Source: three-view drawing plus pictorial views. Frame: mm from the lowest corner of the part. A direction names the side the tool comes from. Give positions to 0.01 mm unless a question says otherwise; leave off trailing zeros. Loops run counter-clockwise (first coordinate to the right, second up) from the corner with the lowest first, then second, coordinate; pieces in that order, holes last. Notation, with made-up numbers: (0, -37.75) - (5, -37.75) arc R18 cw to (5, -21.75) - close; hole circle Ø3 at (89, 86). An arc over 180 degrees is marked (long way). Put each result on its own line as item: value.
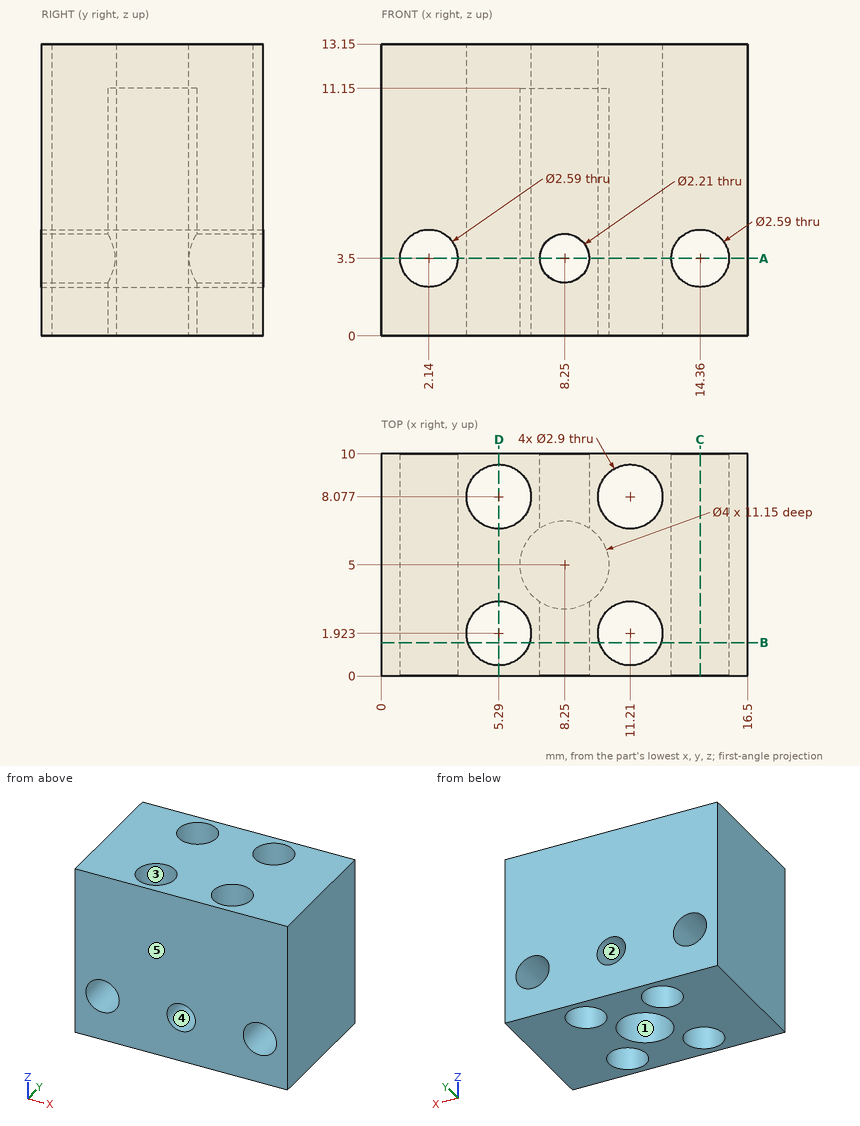
1) Material intervals for line 1 along X through (y, z) = (8, 10.5); line 2 along Y through (x, z) = (11.21, 4.25); line 3 along Z through (x, y) = (8.25, 2.45) (3 decimals), sorted ascending. Write a range as [from, to].
Check result:
line 1: [0, 3.84], [6.74, 9.76], [12.66, 16.5]
line 2: [0, 0.47], [3.37, 6.63], [9.53, 10]
line 3: [0, 2.395], [4.605, 13.15]
2) Section query B-B, the plane y = 1.5. Output: boundary loops of the cut face in (x, z) (3 decimals), plus the area to 3 significant figures.
Check result:
outline: (0, 0) - (3.903, 0) - (3.903, 13.15) - (0, 13.15) - close; (6.677, 0) - (9.823, 0) - (9.823, 13.15) - (6.677, 13.15) - close; (12.597, 0) - (16.5, 0) - (16.5, 13.15) - (12.597, 13.15) - close; hole circle Ø2.59 at (2.14, 3.5); hole circle Ø2.21 at (8.25, 3.5); hole circle Ø2.59 at (14.36, 3.5)
area: 130 mm²
3) Mould query, pull axis Y, two halves, no side actions, for the marked faces 3, 4 and 5. Classes: pulls with the +Y half, pulls with the -Y half, needs draft (parallel to the pull), parting line crosses it, or undercut.
Check result:
face 3: undercut
face 4: needs draft
face 5: pulls with the -Y half
4) Section query A-A, the plane z = 3.5. Output: boundary loops of the cut face in (x, y) (3 decimals), plus the area to 3 significant figures.
Check result:
outline: (0, 0) - (0.845, 0) - (0.845, 10) - (0, 10) - close; (3.435, 0) - (7.145, 0) - (7.145, 3.333) arc R2 cw to (7.145, 6.667) - (7.145, 10) - (3.435, 10) - close; (9.355, 0) - (13.065, 0) - (13.065, 10) - (9.355, 10) - (9.355, 6.667) arc R2 cw to (9.355, 3.333) - close; (15.655, 0) - (16.5, 0) - (16.5, 10) - (15.655, 10) - close; hole circle Ø2.9 at (5.29, 1.923); hole circle Ø2.9 at (5.29, 8.077); hole circle Ø2.9 at (11.21, 1.923); hole circle Ø2.9 at (11.21, 8.077)
area: 60.5 mm²
5) Access query for the marked faces 1 and 2. Directions: +Z, -Z, +X, -X, +Y, -Y. A direction counts if a zero-diameter tool reaches every point of the face in a straight line with its end or side. Return the directions, or none.
Check result:
face 1: -Z
face 2: +Y, -Y
6) Section query C-C, the plane x = 14.36. Output: boundary loops of the cut face in (y, z) (3 decimals).
Check result:
outline: (0, 0) - (10, 0) - (10, 2.205) - (0, 2.205) - close; (0, 4.795) - (10, 4.795) - (10, 13.15) - (0, 13.15) - close
7) Pin query (flat end, axial travel): P1, Ø2, axis at x = 8, y = 5, coming from the -Z side. Return the tip coordinate at first contact, or that it passes through.
Check result:
P1: z = 11.15
8) Section query D-D, the plane x = 5.29. Output: boundary loops of the cut face in (y, z).
Check result:
outline: (0, 0) - (0.47, 0) - (0.47, 13.15) - (0, 13.15) - close; (3.37, 0) - (6.63, 0) - (6.63, 13.15) - (3.37, 13.15) - close; (9.53, 0) - (10, 0) - (10, 13.15) - (9.53, 13.15) - close
